Geometry check sheet. Reference: the model listing, model coordinates, mm. A direction names the side the tool comes from. Round coordinates to 2 decimals unless told otherwise and drop trailing zeros. Loops run counter-clockwise (first coordinate to the right, second up) from the corner with the lowest first, then second, coordinate; pieces in that order, holes last. Notation, with made-up numbers: M 34,-8 L 51,-8 A8 ccw 51,6 Z; hole C 83.25,10 d4. An arc over 180 degrees is marked long. Write item = value, one per line.
Autodesk Inventor part; units mm, degrees
ref_plane "YZ Plane" through (0, 0, 0) normal (1, 0, 0) x (0, 1, 0)
ref_plane "XZ Plane" through (0, 0, 0) normal (0, 1, 0) x (-1, 0, 0)
ref_plane "XY Plane" through (0, 0, 0) normal (0, 0, 1) x (1, 0, 0)
sketch "Sketch1" plane through (0, 0, 0) normal (0, 0, 1) x (1, 0, 0)
  circle A0 centre (0, 0) radius 5
  dimension "d0" = 10
extrude "Extrusion1" add sketch "Sketch1" along normal blind 70
sketch "Sketch2" plane through (0, 0, 70) normal (0, 0, 1) x (1, 0, 0)
  circle A0 centre (0, 0) radius 7.5
  dimension "d3" = 15
extrude "Extrusion2" add sketch "Sketch2" along normal blind 5
fillet "Fillet1" radius 7.25 2 edges at (-5, 0, 70) (-7.5, 0, 70)
sketch "Sketch3" plane through (0, 0, 0) normal (0, 0, -1) x (-1, 0, 0)
  line L0 (27.5, -27.5) -> (-27.5, -27.5)
  line L1 (-27.5, -27.5) -> (-27.5, 27.5)
  line L2 (-27.5, 27.5) -> (27.5, 27.5)
  line L3 (27.5, 27.5) -> (27.5, -27.5)
  line L4 (27.5, -27.5) -> (-27.5, 27.5) construction
  line L5 (-27.5, -27.5) -> (27.5, 27.5) construction
  point P0 (0, 0)
  dimension "d7" = 55
  dimension "d8" = 55
extrude "Extrusion3" add sketch "Sketch3" along normal blind 5
fillet "Fillet2" radius 7.25 1 edges at (-5, 0, 0)
properties part number "Base"
(1) Sectioned sample at A-A on z = 30. Record the cut outline in (x, y), then the cut area to 3 significant figures.
Result set:
outline = C 0,0 d10
area = 78.5 mm2
(2) Material ranges on line 1 along Z through (x, y) = (22.5, -4.5); line 2 along Z through (x, y) = (-6.5, -1); line 3 along Y through (x, z) = (1, 16), recorded low to high. Write a range as from..to.
Result set:
line_1 = -5..0
line_2 = -5..2.74, 69.12..75
line_3 = -4.9..4.9
(3) Sectioned sample at B-B on x = -18. Record the cut outline in (y, z).
Result set:
outline = M -27.5,-5 L 27.5,-5 L 27.5,0 L -27.5,0 Z
(4) Tool access check on faces 1 (the cylindrical face through (-7.493, -0.33, 73.815)), 2 (the flat face through (-27.5, 0, -2)), 3 (the cylindrical face through (-1.08, 4.88, 35.49)). Record the directions out of +Z, -Z, +X, -X, +Y, -Y that give a thin tool (end or side, any length) a straight path to the whole face; none if there is none.
Result set:
face_1 = +Z
face_2 = +Z, -Z, -X, +Y, -Y
face_3 = none
(5) Depth check by flat-ended pin: pin 1 Ø3 at (x, y) = (18.5, -2.5) entering from +Z; pin 2 Ø10 at (x, z) = (11.5, 13.5) entering from +Y; pin 3 Ø5 at (x, z) = (-5.5, 48.5) entering from +Y. Enter the tip coordinate at first touch or a pass-through.
Result set:
pin_1 = 0
pin_2 = through
pin_3 = 4
